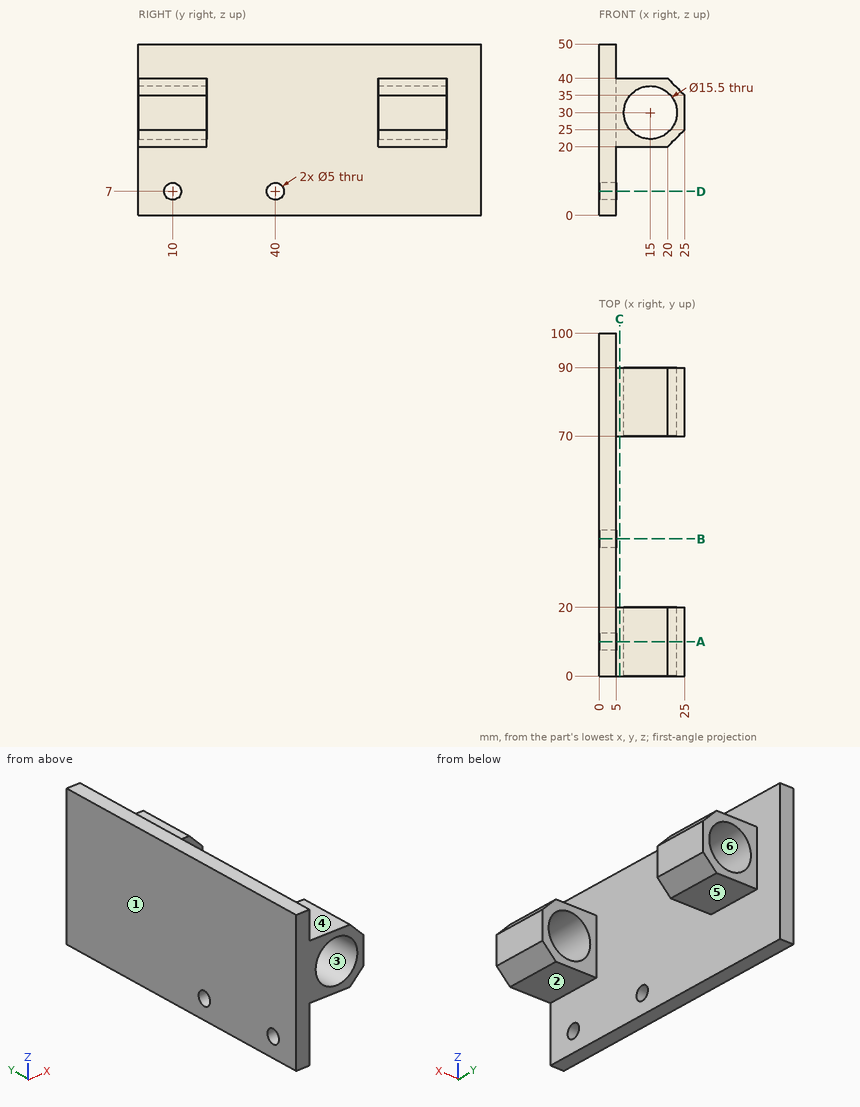
Job drawing, mm, ordinate dimensions from the low corner. One solid piece. A direction names the side the tool comes from. Coordinates: 2 decimals unless noted, no trailing zeros. Loops run counter-clockwise (first coordinate to the right, second up) from the corner with the lowest first, then second, coordinate; pieces in that order, holes last. Notation, with made-up numbers: (28, -31.75) - (67, -31.75) arc R10 ccw to (67, -12.75) - close; hole circle Ø3 at (53, 37.25). An arc over 180 degrees is marked (long way). Answer as a JSON object with one key per item and string values. Group by question number.
(1) Cut at B-B (y = 40). Give the cut face in (x, z).
(2) Two-plate mould, pull along Z, no slides. Class the marked faces 3, 4, 5 and 6: released by +Z, released by -Z, zero draft, split by the parting line, or undercut.
(3) Cut at A-A (y = 10). Give the cut face in (x, z).
(4) Tool access for the marked faces 1 and 2: list every direction of +Z, -Z, +X, -X, +Y, -Y with a clear straight run to the whole face (end or side of a thin tool).
(5) Cut at C-C (x = 6). Give the cut face in (y, z).
(6) Cut at D-D (z = 7). Give the cut face in (x, y).
(7) Flat gauge pins, fed straight in: pin 1 (1 mm diameter, centred on x = 22, z = 28.5, fed in from -Y); pin 2 (4 mm diameter, centred on x = 18, y = 88.5, fed in from +Z); pin 3 (5 mm diameter, centred on y = 51, z = 29, fed in from +X); pin 4 (4.5 mm diameter, centred on x = 13.5, y = 85, fed in from -Z). Where does each tip first touch, or does it go through?
(8) Probe line 1 along Z through (x, y) = (1.55, 10); line 2 along Z through (x, y) = (14.75, 16); line 3 along X through (y, z) = (9, 19). List the from-to ranges inside material, lowest first.
Geometry says:
{
 "1": {"outline": "(0, 0) - (5, 0) - (5, 4.5) - (0, 4.5) - close; (0, 9.5) - (5, 9.5) - (5, 50) - (0, 50) - close"},
 "2": {"face 3": "undercut", "face 4": "released by +Z", "face 5": "released by -Z", "face 6": "undercut"},
 "3": {"outline": "(0, 0) - (5, 0) - (5, 4.5) - (0, 4.5) - close; (0, 9.5) - (5, 9.5) - (5, 20) - (20, 20) - (25, 25) - (25, 35) - (20, 40) - (5, 40) - (5, 50) - (0, 50) - close; hole circle Ø15.5 at (15, 30)"},
 "4": {"face 1": "+Z, -Z, -X, +Y, -Y", "face 2": "-Z, +X, +Y, -Y"},
 "5": {"outline": "(0, 20) - (20, 20) - (20, 40) - (0, 40) - close; (70, 20) - (90, 20) - (90, 40) - (70, 40) - close"},
 "6": {"outline": "(0, 0) - (5, 0) - (5, 7.5) - (0, 7.5) - close; (0, 12.5) - (5, 12.5) - (5, 37.5) - (0, 37.5) - close; (0, 42.5) - (5, 42.5) - (5, 100) - (0, 100) - close"},
 "7": {"pin 1": "passes through", "pin 2": "stops at z = 40", "pin 3": "stops at x = 5", "pin 4": "stops at z = 20"},
 "8": {"line 1": "z = 0 to 4.5, 9.5 to 50", "line 2": "z = 20 to 22.25, 37.75 to 40", "line 3": "x = 0 to 5"}
}
